Part model, mm, in its own coordinate system. A direction names the side the tool comes from. Coordinates: 2 decimals unless noted, no trailing zeros. Write each loop counter-clockwise with the first axis right and the second up, starting at its lowest first coordinate (ties: lowest second). Pieces come first, ordered by that corner, then holes. Notation, with made-up numbers: M 3,37.25 L 60,37.25 A20 ccw 60,52.25 Z; hole C 85.5,39 d5. An arc over 180 degrees is marked long. Use a Markdown table: item, result. Add a question column.
Q1. Slice it at B-B on x = 63.5. Write the cut outline in (y, z) (3 decimals).
Q2. Slice it at C-C on x = -30. Write the cut outline in (y, z), then the cut area to 4 significant figures.
Q3. Mould opens along Y. For faces 1 (the flat face through (0, 96.73, 3)), 2 (the flat face through (2, 30, 6)), 3 (the flat face through (-71, -24.645, 3)) say: released by +Y, released by -Y, zero draft, split by the parting line, or undercut.
Q4. Slice it at D-D on z = 4.65. Count the separate pieces of the cut face and the enclosed holes in it, then the cut area to 3 significant figures.
Q5. Pin check, flat tips, straight feed: pin 1 Ø3 at (y, z) = (-34.5, 2) entering from +X; pin 2 Ø3 at (y, z) = (34.5, 3) entering from -X; pin 3 Ø3 at (x, z) = (-161.5, 2.5) entering from -Y. Stop position of each tip, or through.
Q6. Slice it at A-A on x = -130. Write the cut outline in (y, z) (3 decimals).
Q7. Tool access for faces 4 (the flat face through (-64, -10, 3)), 5 (the flat face through (89, -35, 3)), 6 (the flat face through (95, 94, 3)), 7 (the flat face through (149, 28.73, 3)): list every direction of +Z, -Z, +X, -X, +Y, -Y with a clear straight run to the whole face (end or side of a thin tool).
Q8. Wall check: L1, parallel to Y at x = -70, z = 5.7 (3 decimals); L2, parallel to Y at x = 84, z = 4.6 (3 decimals); L3, parallel to Y at x = -162, z = 1.35. Give the ranges that are in metal, low to high. Write a range as from..to.
from build123d import *

# Parameters (mm, degrees)
BOSS_EXTRU_1_DEPTH      = 6
ESQUISSE3_R             = 8
ESQUISSE3_W             = 6
ESQUISSE3_H             = 10
ESQUISSE3_W_2           = 20
ESQUISSE3_H_2           = 6
ESQUISSE3_W_3           = 60
ESQUISSE3_H_3           = 110
ESQUISSE3_H_4           = 20
ESQUISSE3_W_4           = 8
ESQUISSE3_W_5           = 15
ESQUISSE3_H_5           = 29
ENL_V_MAT_EXTRU_2_DEPTH = 6
ESQUISSE4_R             = 1.5
ENL_V_MAT_EXTRU_3_DEPTH = 6
ESQUISSE5_W             = 456.045253014
ESQUISSE5_H             = 136.228984631
ENL_V_MAT_EXTRU_4_DEPTH = 6
ESQUISSE6_W             = 21
ESQUISSE6_H             = 8
ENL_V_MAT_EXTRU_5_DEPTH = 10


with BuildPart() as part:
    # Esquisse1 → Boss.-Extru.1 (new body)
    with BuildSketch(Plane.XY):
        Polygon((-165, 96.73), (165, 96.73), (165, -18.27), (123, -109.022410436), (-123, -109.022410436), (-165, -18.27), align=None)
    extrude(amount=BOSS_EXTRU_1_DEPTH)

    # Esquisse3 → Enlèv. mat.-Extru.2 (cut)
    with BuildSketch(Plane(origin=(0, 0, 0), x_dir=(-1, 0, 0), z_dir=(0, 0, -1))):
        with Locations((130, -10.145)):
            Circle(ESQUISSE3_R)
        Polygon((165, -3.06), (159, -3.06), (159, 11.73), (39, 11.73), (39, 69.73), (165, 69.73), align=None)
        with Locations((162, 83.23258956)):
            Rectangle(ESQUISSE3_W, ESQUISSE3_H)
        with Locations((-24, -35.02)):
            Rectangle(ESQUISSE3_W_2, ESQUISSE3_H_2)
        with Locations((99, -35.02)):
            Rectangle(ESQUISSE3_W_2, ESQUISSE3_H_2)
        with Locations((-80, 29.355)):
            Rectangle(ESQUISSE3_W_3, ESQUISSE3_H_3)
        with Locations((-162, 72.73)):
            Rectangle(ESQUISSE3_W, ESQUISSE3_H_4)
        with Locations((24, -35.02)):
            Rectangle(ESQUISSE3_W_2, ESQUISSE3_H_2)
        with Locations((-162, 36.44)):
            Rectangle(ESQUISSE3_W, ESQUISSE3_H_4)
        with Locations((-162, 0.15)):
            Rectangle(ESQUISSE3_W, ESQUISSE3_H_4)
        with Locations((105, 93.73)):
            Rectangle(ESQUISSE3_W_2, ESQUISSE3_H_2)
        with Locations((-35, 93.73)):
            Rectangle(ESQUISSE3_W_2, ESQUISSE3_H_2)
        with Locations((35, 93.73)):
            Rectangle(ESQUISSE3_W_2, ESQUISSE3_H_2)
        with Locations((-105, 93.73)):
            Rectangle(ESQUISSE3_W_2, ESQUISSE3_H_2)
        with Locations((100.5, -10.145)):
            Rectangle(ESQUISSE3_W_4, ESQUISSE3_H_4)
        with Locations((-99, -35.02)):
            Rectangle(ESQUISSE3_W_2, ESQUISSE3_H_2)
        with Locations((71.5, -10.145)):
            Rectangle(ESQUISSE3_W_5, ESQUISSE3_H_5)
    extrude(amount=-ENL_V_MAT_EXTRU_2_DEPTH, mode=Mode.SUBTRACT)

    # Esquisse4 → Enlèv. mat.-Extru.3 (cut)
    with BuildSketch(Plane(origin=(0, 0, 0), x_dir=(-1, 0, 0), z_dir=(0, 0, -1))):
        with Locations((114, -35.02)):
            Circle(ESQUISSE4_R)
        with Locations((162, 73.98258956)):
            Circle(ESQUISSE4_R)
        with Locations((84, -35.02)):
            Circle(ESQUISSE4_R)
        with Locations((39, -35.02)):
            Circle(ESQUISSE4_R)
        with Locations((162, -6.46)):
            Circle(ESQUISSE4_R)
        with Locations((9, -35.02)):
            Circle(ESQUISSE4_R)
        with Locations((-9, -35.02)):
            Circle(ESQUISSE4_R)
        with Locations((-39, -35.02)):
            Circle(ESQUISSE4_R)
        with Locations((-84, -35.02)):
            Circle(ESQUISSE4_R)
        with Locations((120, 93.73)):
            Circle(ESQUISSE4_R)
        with Locations((-114, -35.02)):
            Circle(ESQUISSE4_R)
        with Locations((90, 93.73)):
            Circle(ESQUISSE4_R)
        with Locations((50, 93.73)):
            Circle(ESQUISSE4_R)
        with Locations((20, 93.73)):
            Circle(ESQUISSE4_R)
        with Locations((-162, 18.29)):
            Circle(ESQUISSE4_R)
        with Locations((-162, 54.585)):
            Circle(ESQUISSE4_R)
        with Locations((-20, 93.73)):
            Circle(ESQUISSE4_R)
        with Locations((-50, 93.73)):
            Circle(ESQUISSE4_R)
        with Locations((-90, 93.73)):
            Circle(ESQUISSE4_R)
        with Locations((-120, 93.73)):
            Circle(ESQUISSE4_R)
    extrude(amount=-ENL_V_MAT_EXTRU_3_DEPTH, mode=Mode.SUBTRACT)

    # Esquisse5 → Enlèv. mat.-Extru.4 (cut)
    with BuildSketch(Plane(origin=(0, 0, 0), x_dir=(-1, 0, 0), z_dir=(0, 0, -1))):
        with Locations((-18.307092018, -106.134492316)):
            Rectangle(ESQUISSE5_W, ESQUISSE5_H)
    extrude(amount=-ENL_V_MAT_EXTRU_4_DEPTH, mode=Mode.SUBTRACT)

    # Esquisse6 → Enlèv. mat.-Extru.5 (cut)
    with BuildSketch(Plane(origin=(0, 0, 0), x_dir=(-1, 0, 0), z_dir=(0, 0, -1))):
        with Locations((-148.5, 32.73)):
            Rectangle(ESQUISSE6_W, ESQUISSE6_H)
    extrude(amount=-ENL_V_MAT_EXTRU_5_DEPTH, mode=Mode.SUBTRACT)


solid = part.part
Recorded:
| question | item | result |
|---|---|---|
| 1 | outline | M -38.02,0 L -25.645,0 L -25.645,6 L -38.02,6 Z; M 84.355,0 L 96.73,0 L 96.73,6 L 84.355,6 Z |
| 2 | outline | M -32.02,0 L 90.73,0 L 90.73,6 L -32.02,6 Z |
| 2 | area | 736.5 mm² |
| 3 | face 1 | released by +Y |
| 3 | face 2 | zero draft |
| 3 | face 3 | undercut |
| 4 | separate pieces | 1 |
| 4 | enclosed holes | 24 |
| 4 | area | 27,800 mm² |
| 5 | pin 1 | x = 158.18 |
| 5 | pin 2 | x = -39 |
| 5 | pin 3 | y = -29.07 |
| 6 | outline | M -38.02,0 L -18.145,0 L -18.145,6 L -38.02,6 Z; M -2.145,0 L 11.73,0 L 11.73,6 L -2.145,6 Z; M 69.73,0 L 96.73,0 L 96.73,6 L 69.73,6 Z |
| 7 | face 4 | +Z, -Z |
| 7 | face 5 | +Z, -Z, -Y |
| 7 | face 6 | +Z, -Z, +Y |
| 7 | face 7 | +Z, -Z, +X |
| 8 | L1 | -38.02..-24.645, 4.355..11.73, 69.73..96.73 |
| 8 | L2 | -38.02..-36.52, -33.52..-25.645, 84.355..96.73 |
| 8 | L3 | -24.75..-7.96, -4.96..-3.06, 69.73..72.48, 75.48..78.23, 88.23..96.73 |
